Read the model definition and answer for the solid it produces. Units are mm, in the model's axes. A direction names the side the tool comes from. Give positions to 0.01 mm unless a question says otherwise; leave off trailing zeros. Loops run counter-clockwise (first coordinate to the right, second up) from the corner with the lowest first, then second, coordinate; pieces in that order, holes last. Notation, with made-up numbers: (67.25, -6.75) - (102.25, -6.75) arc R14 cw to (102.25, 13.25) - close; hole circle Ø10 at (-3.5, -39). An arc over 180 degrees is marked (long way). Use a Markdown table: item, result. Add a question column.
Item 1: A cutting plane is placed at A-A (z = 13.5). Determine the outline of the cut face in (x, y).
Item 2: Which of the six approach directions +Z, -Z, +X, -X, +Y, -Y give full straight-line access (tool end or side, diameter ignored) to faces 4 (the face through (0.1, 5.45, -15.67)), 5 (the face through (2, 3.62, 15)), 6 (the face through (-10.77, 4.1, -1.9)), 7 (the face through (-2, 3.62, -16))?
Item 3: Consider probe 1 along Z at (x, y) = (0, 1.55); probe 2 along Z at (x, y) = (-1.5, 6.5); probe 3 along X at (y, z) = (3.25, 7). Determine where each line is inside the solid, lowest interval first. Write a range as [from, to].
Item 4: Each of these flat-tipped pins is pushed along its axis until it touches: P1, Ø2, axis at x = 3.5, z = 13.5, coming from the +Y side; P2, Ø3, axis at y = 2, z = -9, coming from the -X side; P3, Ø6, axis at x = -0.5, z = -12.5, coming from the -Y side. Where does it stop, or does it pass through?
Item 5: For a pull along Z with two mould halves and no side action, classify faces 1 (the face through (-9, 7.239, -7)), 2 (the face through (-6.977, 5.455, 12.085)), 3 (the face through (-0.1, 1.84, 15.67)) as +Z half, -Z half, draft (parallel to the pull), parting line (faces both ways), or undercut.
Item 6: A cutting plane is placed at B-B (x = 0). Determine the outline of the cut face in (y, z), plus the area to 3 significant figures.
Item 7: A cutting plane is placed at D-D (z = -5). Determine the outline of the cut face in (x, y), plus the area to 3 significant figures.
Item 8: A cutting plane is placed at C-C (z = 0). Determine the outline of the cut face in (x, y).
from build123d import *

# Parameters (mm, degrees)
SKETCH1_R         = 16.891
EXTRUDE1_DEPTH    = 7.239
SKETCH2_R         = 10.9347
EXTRUDE2_DEPTH    = 25.960266084
SKETCH3_R         = 10.9347
SKETCH3_R_2       = 9.9568
EXTRUDE3_DEPTH    = 1.0414
SKETCH4_R         = 2.1844
EXTRUDE4_DEPTH    = 25.960266084
CIRPATTERN1_COUNT = 6
EXTRUDE6_DEPTH    = 25.960266084
EXTRUDE7_DEPTH    = 3.6195
EXTRUDE8_DEPTH    = 3.6195
EXTRUDE12_DEPTH   = 25.160143672


with BuildPart() as part:
    # Sketch1 → Extrude1 (new body)
    with BuildSketch(Plane(origin=(0, 0, 0), x_dir=(1, 0, 0), z_dir=(0, 1, 0))):
        with Locations(Location((0, 0, 0), (0, 0, 270))):
            Circle(SKETCH1_R)
    extrude(amount=EXTRUDE1_DEPTH)

    # Sketch2 → Extrude2 (cut, through all)
    with BuildSketch(Plane.XZ):
        with Locations(Location((0, 0, 0), (0, 0, 270))):
            Circle(SKETCH2_R)
    extrude(amount=-EXTRUDE2_DEPTH, mode=Mode.SUBTRACT)

    # Sketch3 → Extrude3 (add)
    with BuildSketch(Plane.XZ):
        with Locations(Location((0, 0, 0), (0, 0, 270))):
            Circle(SKETCH3_R)
        with Locations(Location((0, 0, 0), (0, 0, 270))):
            Circle(SKETCH3_R_2, mode=Mode.SUBTRACT)
    extrude(amount=-EXTRUDE3_DEPTH)

    # Sketch4 → Extrude4 (cut, through all)
    with BuildSketch(Plane(origin=(0, 7.239, 0), x_dir=(1, 0, 0), z_dir=(0, 1, 0))):
        with Locations(Location((0, 13.4874, 0), (0, 0, 270))):
            Circle(SKETCH4_R)
    extrude4 = extrude(amount=-EXTRUDE4_DEPTH, mode=Mode.SUBTRACT)

    # CirPattern1: Extrude4 ×6 about axis
    cirpattern1_axis = Axis((0, 0, 0), (0, 1, 0))
    for i in range(1, CIRPATTERN1_COUNT):
        add(extrude4.rotate(cirpattern1_axis, i * 360 / CIRPATTERN1_COUNT), mode=Mode.SUBTRACT)

    # Sketch7 → Extrude6 (cut, through all)
    with BuildSketch(Plane(origin=(0, 7.239, 0), x_dir=(1, 0, 0), z_dir=(0, 1, 0))):
        Polygon((0, 0), (16.891, 29.256070191), (16.891, -29.256070191), align=None)
    extrude(amount=-EXTRUDE6_DEPTH, mode=Mode.SUBTRACT)

    # Sketch8 → Extrude7 (cut)
    with BuildSketch(Plane(origin=(0, 7.239, 0), x_dir=(1, 0, 0), z_dir=(0, 1, 0))):
        Polygon((0, 0), (9.752023397, -16.891), (-9.752023397, -16.891), align=None)
    extrude(amount=-EXTRUDE7_DEPTH, mode=Mode.SUBTRACT)

    # Sketch9 → Extrude8 (cut)
    with BuildSketch(Plane.XZ):
        Polygon((0, 0), (9.752023397, -16.891), (-9.752023397, -16.891), align=None)
    extrude(amount=-EXTRUDE8_DEPTH, mode=Mode.SUBTRACT)

    # Sketch13 → Extrude12 (cut, through all)
    with BuildSketch(Plane(origin=(0, 3.6195, 0), x_dir=(1, 0, 0), z_dir=(0, 1, 0))):
        Polygon((0.998562219, 10.889009945), (6.992650397, 12.111625767), (4.9784, -8.62284174), align=None)
    extrude(amount=EXTRUDE12_DEPTH, mode=Mode.SUBTRACT)


solid = part.part
Geometry says:
| question | item | result |
|---|---|---|
| 1 | outline | (-10.15, 0) - (-2.18, 0) - (-2.18, 3.62) - (-7.79, 3.62) - (-7.79, 7.24) - (-10.15, 7.24) - close; (2.18, 0) - (7.79, 0) - (7.79, 3.62) - (2.18, 3.62) - close |
| 2 | face 4 | +Y, -Y |
| 2 | face 5 | +Z, +X, +Y |
| 2 | face 6 | +Y |
| 2 | face 7 | -Z, +X, -Y |
| 3 | probe 1 | [10.93, 11.3], [15.67, 16.89] |
| 3 | probe 2 | [-16.82, -15.08], [-11.9, -10.83] |
| 3 | probe 3 | [-15.37, -13.85], [-9.51, -8.4] |
| 4 | P1 | y = 3.62 |
| 4 | P2 | x = -15.13 |
| 4 | P3 | y = 3.62 |
| 5 | face 1 | draft |
| 5 | face 2 | +Z half |
| 5 | face 3 | undercut |
| 6 | outline | (0, 9.96) - (1.04, 9.96) - (1.04, 10.93) - (3.62, 10.93) - (3.62, 11.3) - (0, 11.3) - close; (0, 15.67) - (3.62, 15.67) - (3.62, 16.89) - (0, 16.89) - close; (3.62, -16.89) - (7.24, -16.89) - (7.24, -15.67) - (3.62, -15.67) - close; (3.62, -11.3) - (7.24, -11.3) - (7.24, -10.93) - (3.62, -10.93) - close |
| 6 | area | 12.5 mm² |
| 7 | outline | (-16.13, 0) - (-13, 0) - (-13, 7.24) - (-16.13, 7.24) - close; (-10.36, 0) - (-8.61, 0) - (-8.61, 1.04) - (-9.72, 1.04) - (-9.72, 7.24) - (-10.36, 7.24) - close |
| 7 | area | 28.5 mm² |
| 8 | outline | (-16.89, 0) - (-9.96, 0) - (-9.96, 1.04) - (-10.93, 1.04) - (-10.93, 7.24) - (-16.89, 7.24) - close |
